Geometry check sheet. Reference: the model listing, model coordinates, mm. Face numbers are marked on the shaded views. Round coordinates to 2 decimals unless told otherwise and drop trailing zeros. Order: outer loops, then holes, each group sorted by start corner. A loop starts at its lowest first (then second) coordinate and runs counter-clockwise, first axis right, second up.
(1) Sectioned sample at A-A (x = -72.4). Record the boundary of the cut face in (y, z).
(2) Sectioned sample at D-D (y = -13). Record the boundary of the cut face in (x, z), plus the area to 3 significant figures.
(3) Sectioned sample at C-C (x = -37.5). Record the boundary of the cut face in (y, z).
(4) Sectioned sample at B-B (y = 0). Record the boundary of the cut face in (x, z), plus the area to 3 significant figures.
(5) Material ranges on line 1 along Y through (x, z) = (-72.4, 1.25); line 2 along X through (y, z) = (-2.5, 0.4); line 3 along Y through (x, z) = (-73, 1.85), recorded low to high.
(6) Release check for a two-part mould opening along Z. For the marked faces 1 and 2 record: +Z half, -Z half, draft (parallel to the pull), parting line (faces both ways), or undercut.
(7) Go/stop test with flat-tipped pins: pin 1 (0.6 mm diameter, centred on x = -23, z = 1, fed in from -Y); pin 2 (2.5 mm diameter, centred on x = -72.4, y = 5, fed in from +Z); pin 3 (1 mm diameter, centred on x = -34, z = 1.5, fed in from -Y); pin 4 (1 mm diameter, centred on x = -13, z = 1, fed in from +Y). Record where each tip stops, or that it passes through.
from build123d import *

# Parameters (mm, degrees)
SKETCH1_R      = 2
EXTRUDE1_DEPTH = 2
SKETCH2_R      = 1.5
EXTRUDE2_DEPTH = 2
EXTRUDE3_DEPTH = 2
EXTRUDE4_DEPTH = 2
SKETCH5_R      = 14.5
EXTRUDE5_DEPTH = 2


with BuildPart() as part:
    # Sketch1 → Extrude1 (new body)
    with BuildSketch(Plane.XY):
        with BuildLine():
            Line((1.27220287, -11.932371929), (-27.5, -15))
            Line((-27.5, -15), (-29.540064206, -15))
            ThreePointArc((-29.540064206, -15), (-42, -19.5), (-54.459935794, -15))
            Line((-54.459935794, -15), (-77.8, -15))
            Line((-77.8, -15), (-77.8, 15))
            Line((-77.8, 15), (-54.459935794, 15))
            ThreePointArc((-54.459935794, 15), (-42, 19.5), (-29.540064206, 15))
            Line((-29.540064206, 15), (-27.5, 15))
            Line((-27.5, 15), (1.27220287, 11.932371929))
            ThreePointArc((1.27220287, 11.932371929), (12, 0), (1.27220287, -11.932371929))
        make_face()
        Circle(SKETCH1_R, mode=Mode.SUBTRACT)
    extrude(amount=EXTRUDE1_DEPTH)

    # Sketch2 → Extrude2 (cut)
    with BuildSketch(Plane.XY.offset(2)):
        with Locations((-23.2, 5)):
            Circle(SKETCH2_R)
        with Locations((-72.4, 5)):
            Circle(SKETCH2_R)
        with Locations(Location((-23.2, -5, 0), (0, 0, 180))):
            Circle(SKETCH2_R)
        with Locations(Location((-72.4, -5, 0), (0, 0, 180))):
            Circle(SKETCH2_R)
    extrude(amount=-EXTRUDE2_DEPTH, mode=Mode.SUBTRACT)

    # Sketch3 → Extrude3 (cut)
    with BuildSketch(Plane.XY.offset(2)):
        with BuildLine():
            Line((-13.5, 5), (-11.5, 5))
            ThreePointArc((-11.5, 5), (-10.792893219, 4.707106781), (-10.5, 4))
            Line((-10.5, 4), (-10.5, -4))
            ThreePointArc((-10.5, -4), (-10.792893219, -4.707106781), (-11.5, -5))
            Line((-11.5, -5), (-13.5, -5))
            ThreePointArc((-13.5, -5), (-14.207106781, -4.707106781), (-14.5, -4))
            Line((-14.5, -4), (-14.5, 4))
            ThreePointArc((-14.5, 4), (-14.207106781, 4.707106781), (-13.5, 5))
        make_face()
    extrude(amount=-EXTRUDE3_DEPTH, mode=Mode.SUBTRACT)

    # Sketch4 → Extrude4 (cut)
    with BuildSketch(Plane.XY.offset(2)):
        Polygon((-27.5, -1), (-27.5, -10), (-67.8, -10), (-67.8, -1), (-75.8, -1), (-75.8, 1), (-67.8, 1), (-67.8, 10), (-27.5, 10), (-27.5, 1), (-19.5, 1), (-19.5, -1), align=None)
    extrude(amount=-EXTRUDE4_DEPTH, mode=Mode.SUBTRACT)

    # Sketch5 → Extrude5 (cut)
    with BuildSketch(Plane.XY.offset(2)):
        with Locations((-42, 0)):
            Circle(SKETCH5_R)
    extrude(amount=-EXTRUDE5_DEPTH, mode=Mode.SUBTRACT)


solid = part.part
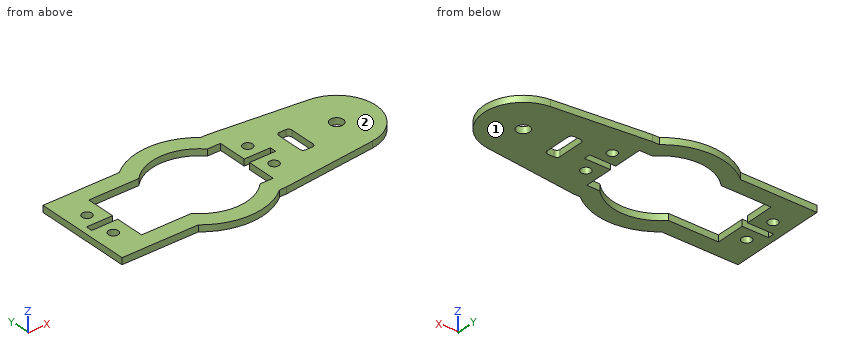
Answer below:
1. outline: (-15, 0) - (-6.5, 0) - (-6.5, 2) - (-15, 2) - close; (-3.5, 0) - (-1, 0) - (-1, 2) - (-3.5, 2) - close; (1, 0) - (3.5, 0) - (3.5, 2) - (1, 2) - close; (6.5, 0) - (15, 0) - (15, 2) - (6.5, 2) - close
2. outline: (-77.8, 0) - (-48.42, 0) - (-48.42, 2) - (-77.8, 2) - close; (-35.58, 0) - (-8.74, 0) - (-8.74, 2) - (-35.58, 2) - close
2. area: 112 mm2
3. outline: (-18.97, 0) - (-13.78, 0) - (-13.78, 2) - (-18.97, 2) - close; (13.78, 0) - (18.97, 0) - (18.97, 2) - (13.78, 2) - close
4. outline: (-77.8, 0) - (-75.8, 0) - (-75.8, 2) - (-77.8, 2) - close; (-19.5, 0) - (-14.5, 0) - (-14.5, 2) - (-19.5, 2) - close; (-10.5, 0) - (-2, 0) - (-2, 2) - (-10.5, 2) - close; (2, 0) - (12, 0) - (12, 2) - (2, 2) - close
4. area: 51.0 mm2
5. line 1: y = -15 to -6.5, -3.5 to -1, 1 to 3.5, 6.5 to 15
5. line 2: x = -77.8 to -67.8, -27.5 to -14.5, -10.5 to 11.74
5. line 3: y = -15 to -6.37, -3.63 to -1, 1 to 3.63, 6.37 to 15
6. face 1: -Z half
6. face 2: +Z half
7. pin 1: stops at y = -14.55
7. pin 2: passes through
7. pin 3: stops at y = -18
7. pin 4: stops at y = 13.51
